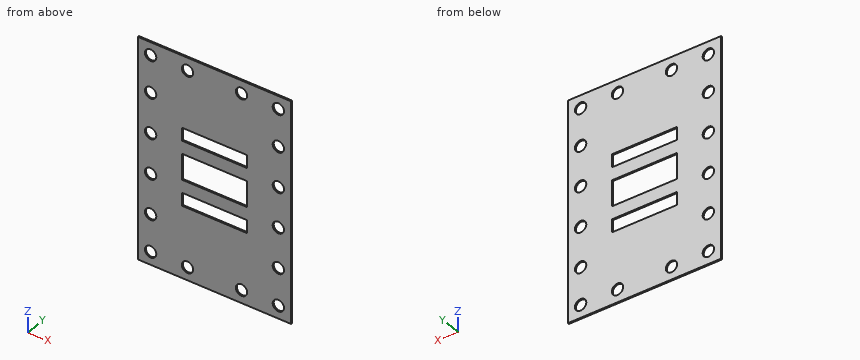
Autodesk Inventor part; units mm, degrees
ref_plane "YZ Plane" through (0, 0, 0) normal (1, 0, 0) x (0, 1, 0)
ref_plane "XZ Plane" through (0, 0, 0) normal (0, 1, 0) x (-1, 0, 0)
ref_plane "XY Plane" through (0, 0, 0) normal (0, 0, 1) x (1, 0, 0)
sketch "Sketch1" plane through (0, 0, 0) normal (0, 1, 0) x (-1, 0, 0)
  line L0 (0, 0) -> (-54, 0)
  line L1 (-54, 0) -> (-54, -77)
  line L2 (-54, -77) -> (0, -77)
  line L3 (0, -77) -> (0, 0)
  line L4 (-4.5, -4.5) -> (-49.5, -4.5) construction
  line L5 (-49.5, -4.5) -> (-49.5, -72.5) construction
  line L6 (-49.5, -72.5) -> (-4.5, -72.5) construction
  line L7 (-4.5, -72.5) -> (-4.5, -4.5) construction
  circle A0 centre (-4.5, -4.5) radius 2
  circle A1 centre (-17.5, -4.5) radius 2
  circle A2 centre (-49.5, -4.5) radius 2
  circle A3 centre (-49.5, -17.5) radius 2
  circle A4 centre (-49.5, -31.5) radius 2
  circle A5 centre (-49.5, -45.5) radius 2
  circle A6 centre (-49.5, -59.5) radius 2
  circle A7 centre (-49.5, -72.5) radius 2
  circle A8 centre (-36.5, -72.5) radius 2
  circle A9 centre (-17.5, -72.5) radius 2
  circle A10 centre (-4.5, -72.5) radius 2
  circle A11 centre (-4.5, -59.5) radius 2
  circle A12 centre (-4.5, -45.5) radius 2
  circle A13 centre (-4.5, -31.5) radius 2
  circle A14 centre (-4.5, -17.5) radius 2
  circle A15 centre (-36.5, -4.5) radius 2
  dimension "d0" = 54
  dimension "d1" = 77
  dimension "d2" = 4
  dimension "d3" = 4
  dimension "d5" = 4
  dimension "d6" = 4
  dimension "d7" = 4
  dimension "d8" = 4
  dimension "d9" = 4
  dimension "d10" = 4
  dimension "d11" = 4
  dimension "d12" = 4
  dimension "d13" = 4
  dimension "d14" = 4
  dimension "d15" = 4
  dimension "d16" = 4
  dimension "d17" = 4
  dimension "d18" = 4.5
  dimension "d20" = 4.5
  dimension "d21" = 4.5
  dimension "d22" = 4.5
  dimension "d23" = 13
  dimension "d27" = 14
  dimension "d28" = 14
  dimension "d29" = 14
  dimension "d30" = 4.5
  dimension "d31" = 4
  dimension "d32" = 13
  dimension "d33" = 19
  dimension "d34" = 13
  dimension "d35" = 14
  dimension "d36" = 14
  dimension "d37" = 14
  dimension "d38" = 13
  dimension "d39" = 19
extrude "Extrusion1" add sketch "Sketch1" along normal blind 0.5
sketch "Sketch2" plane through (0, 0.5, 0) normal (0, 1, 0) x (1, 0, 0)
  line L0 (15.5, 47.5) -> (38.5, 47.5)
  line L1 (38.5, 47.5) -> (38.5, 52)
  line L2 (38.5, 52) -> (15.5, 52)
  line L3 (15.5, 52) -> (15.5, 47.5)
  line L4 (27, 0) -> (27, 77) construction
  line L5 (54, 0) -> (54, 77)
  line L6 (0, 38.5) -> (54, 38.5) construction
  line L7 (54, 77) -> (0, 77)
  line L8 (15.5, 34) -> (38.5, 34)
  line L9 (38.5, 34) -> (38.5, 43)
  line L10 (38.5, 43) -> (15.5, 43)
  line L11 (15.5, 43) -> (15.5, 34)
  line L12 (15.5, 25) -> (38.5, 25)
  line L13 (38.5, 25) -> (38.5, 29.5)
  line L14 (38.5, 29.5) -> (15.5, 29.5)
  line L15 (15.5, 29.5) -> (15.5, 25)
  circle A0 centre (4.5, 45.5) radius 2
  circle A1 centre (4.5, 31.5) radius 2
  point P0 (0, 0)
  point P1 (15.5, 38.5)
  point P2 (27, 43)
  point P3 (27, 47.5)
  point P4 (27, 29.5)
  dimension "d42" = 27
  dimension "d43" = 38.5
  dimension "d47" = 9
  dimension "d48" = 23
  dimension "d49" = 4.5
  dimension "d50" = 4.5
  dimension "d51" = 23
  dimension "d52" = 4.5
  dimension "d53" = 4.5
extrude "Extrusion2" cut sketch "Sketch2" against normal through all contours L3 L2 L1 L0 | L11 L10 L9 L8 | L15 L14 L13 L12
properties part number "1-33"
CAD build for the part. Positions are in the model's coordinates, mm. Coordinates: 2 decimals unless noted, no trailing zeros. Order: outer loops, then holes, each group sorted by start corner. A loop starts at its lowest first (then second) coordinate and runs counter-clockwise, first axis right, second up.
Item 1: Band-saw the part on A-A on z = -17.5. List the corners of the cut face in (x, y), plus the area to 3 significant figures.
Check sheet entries:
outline: (0, 0) - (2.5, 0) - (2.5, 0.5) - (0, 0.5) - close; (6.5, 0) - (47.5, 0) - (47.5, 0.5) - (6.5, 0.5) - close; (51.5, 0) - (54, 0) - (54, 0.5) - (51.5, 0.5) - close
area: 23.0 mm2
Item 2: Drill centre lines: L1, parallel to Z at x = 28, y = 0.45; L2, parallel to Z at x = 36.5, y = 0.45; L3, parallel to Z at x = 16.5, y = 0.15. Where is each one in solid material? Low to high.
Check sheet entries:
L1: z = -77 to -52, -47.5 to -43, -34 to -29.5, -25 to 0
L2: z = -77 to -74.5, -70.5 to -52, -47.5 to -43, -34 to -29.5, -25 to -6.5, -2.5 to 0
L3: z = -77 to -74.23, -70.77 to -52, -47.5 to -43, -34 to -29.5, -25 to -6.23, -2.77 to 0
Item 3: Band-saw the part on C-C on x = 4.5. List the corners of the cut face in (y, z).
Check sheet entries:
outline: (0, -77) - (0.5, -77) - (0.5, -74.5) - (0, -74.5) - close; (0, -70.5) - (0.5, -70.5) - (0.5, -61.5) - (0, -61.5) - close; (0, -57.5) - (0.5, -57.5) - (0.5, -47.5) - (0, -47.5) - close; (0, -43.5) - (0.5, -43.5) - (0.5, -33.5) - (0, -33.5) - close; (0, -29.5) - (0.5, -29.5) - (0.5, -19.5) - (0, -19.5) - close; (0, -15.5) - (0.5, -15.5) - (0.5, -6.5) - (0, -6.5) - close; (0, -2.5) - (0.5, -2.5) - (0.5, 0) - (0, 0) - close
Item 4: Band-saw the part on D-D on y = 0.3. Give the number of separate pieces and of enclosed holes in the cut face, plus the area to 3 significant figures.
Check sheet entries:
separate pieces: 1
enclosed holes: 19
area: 3,540 mm2
Item 5: Pin check, flat tip, straight feed: pin 1 Ø3 at (x, z) = (49.5, -45.5) entering from +Y. Stop position of the tip, or through.
Check sheet entries:
pin 1: passes through
Item 6: Band-saw the part on B-B on z = -35.5. List the corners of the cut face in (x, y).
Check sheet entries:
outline: (0, 0) - (15.5, 0) - (15.5, 0.5) - (0, 0.5) - close; (38.5, 0) - (54, 0) - (54, 0.5) - (38.5, 0.5) - close
